Part model, mm, in its own coordinate system. A direction names the side the tool comes from. Give positions to 0.01 mm unless a question says otherwise; leave off trailing zeros. Order: outer loops, then holes, each group sorted by start corner. A loop starts at its lowest first (then second) coordinate and runs counter-clockwise, first axis right, second up. Notation, with made-up numbers: (39, 52) -> (54, 52) arc R11 ccw to (54, 57) -> close; hole circle Ø5 at (36.5, 85). An arc over 180 degrees is marked (long way). Write item = value, one per line. Start each with the question number.
Item 1: Flat gauge pins, fed straight in: P1, Ø4.5, axis at x = 0, y = 0, coming from the +Z side; P2, Ø8, axis at x = 242.5, z = 77, coming from the -Y side. Where does each tip first touch, or does it go through?
Item 2: Drill centre lines: line 1 along Z through (x, y) = (-242.5, -0.25); line 2 along X through (y, z) = (0, 96.25); line 3 along X through (y, z) = (-1.5, 77). Where is each one in solid material? Low to high.
Item 3: Band-saw the part on A-A on z = 52. Write the cut outline in (x, y), plus the area to 3 significant figures.
Item 4: Tool access for faces 4 (the face through (-3, -7.5, 49)), 5 (the face through (-237.7, 4.5, 25)), 6 (the face through (242, -3.5, 51)), 7 (the face through (-250, 2, 49)), 8 (the face through (-242, -3.233, 51)): list every direction of +Z, -Z, +X, -X, +Y, -Y with a clear straight run to the whole face (end or side of a thin tool).
Item 5: Pull direction X, two halves, no side cores. Call faces 1 (the face through (250, 2, 49)), 2 (the face through (3, 7.5, 49)), 3 (the face through (-242.6, 1.5, 73.6)): +X half, -X half, draft (parallel to the pull), parting line (faces both ways), or undercut.
Solid Edge part; units mm, degrees
sketch "Sketch1" plane through (0, 0, 0) normal (0, 0, 1) x (1, 0, 0)
  line L0 (-250, -7.5) -> (250, -7.5)
  line L1 (250, -7.5) -> (250, 7.5)
  line L2 (250, 7.5) -> (-250, 7.5)
  line L3 (-250, 7.5) -> (-250, -7.5)
extrude "Protrusion1" add sketch "Sketch1" along normal blind 100
sketch "Sketch2" plane through (0, 0, 100) normal (0, 0, 1) x (-1, 0, 0)
  line L0 (250, 7.5) -> (234, 7.5)
  line L1 (234, 7.5) -> (234, 3.2333)
  line L2 (234, 3.2333) -> (250, 3.2333)
  line L3 (250, 3.2333) -> (250, 7.5)
  line L4 (-250, 7.5) -> (-250, 3.5)
  line L5 (-250, 3.5) -> (-234, 3.5)
  line L6 (-234, 3.5) -> (-234, 7.5)
  line L7 (-234, 7.5) -> (-250, 7.5)
extrude "Cutout1" cut sketch "Sketch2" against normal up to next
sketch "Sketch3" plane through (242.5, -3.5, 50) normal (0, -1, 0) x (0, 0, 1)
  circle A0 centre (27, 0) radius 3.1
  circle A1 centre (-27, 0) radius 3.1
  dimension "D1" = 27
extrude "Cutout2" cut sketch "Sketch3" against normal up to next
sketch "Sketch4" plane through (0, 7.5, 50) normal (0, 1, 0) x (-1, 0, 0)
  circle A0 centre (-242.5, -27) radius 5.2
  circle A1 centre (-242.5, 27) radius 5.2
extrude "ExtrudedCutout_3" cut sketch "Sketch4" against normal blind 6
mirror "Mirror1" about plane through (0, 0, 0) normal (1, 0, 0) of "Cutout2", "ExtrudedCutout_3"
hole "Hole_9" at (0, 7.5, 30) direction (0, -1, 0) diameter 4.917 end up to next thread major 6 thread length 15
hole "Hole1" at (-150, 7.5, 30) direction (0, -1, 0) diameter 4.917 end up to next thread major 6 thread length 15
hole "Hole2" at (150, 7.5, 30) direction (0, -1, 0) diameter 4.917 end up to next thread major 6 thread length 15
hole "Hole_15" at (0, 0, 100) direction (0, 0, -1) diameter 4.917 depth 14 thread major 6 thread length 12
hole "Hole3" at (150, 0, 100) direction (0, 0, -1) diameter 4.917 depth 14 thread major 6 thread length 12
hole "Hole4" at (-150, 0, 100) direction (0, 0, -1) diameter 4.917 depth 14 thread major 6 thread length 12
Values found:
q1.P1 = 86
q1.P2 = -3.5
q2.line_1 = 0 to 19.9, 26.1 to 73.9, 80.1 to 100
q2.line_2 = -250 to -152.46, -147.54 to -2.46, 2.46 to 147.54, 152.46 to 250
q2.line_3 = -250 to -245.6, -239.4 to 239.4, 245.6 to 250
q3.outline = (-250, -3.23) -> (-234, -3.23) -> (-234, -7.5) -> (234, -7.5) -> (234, -3.5) -> (250, -3.5) -> (250, 7.5) -> (-250, 7.5) -> close
q3.area = 7,370 mm^2
q4.face_4 = +Z, -Z, +X, -X, -Y
q4.face_5 = +Y
q4.face_6 = +Z, -Z, +X, -Y
q4.face_7 = +Z, -Z, -X, +Y, -Y
q4.face_8 = +Z, -Z, -X, -Y
q5.face_1 = +X half
q5.face_2 = draft
q5.face_3 = undercut
